Verification items for the finished model (mm, model axes). Give positions to 0.01 mm unless a question says otherwise; leave off trailing zeros. Write each loop counter-clockwise with the first axis right and the second up, starting at its lowest first coordinate (ties: lowest second). Pieces come first, ordered by that corner, then holes.
from build123d import *

# Parameters (mm, degrees)
PAD012_DEPTH = 110
BOX_W        = 174
BOX_H        = 120
BOX_DEPTH    = 10


with BuildPart() as pad012:
    # Sketch015 → Pad012 (new body)
    with BuildSketch(Plane.XZ.offset(-110)):
        Polygon((10, 12.723166), (9.966702, 8.484643), (4.563902, 8.484643), (4.5972, 2), (175.457199, 2.027261), (175.44223, 8.564159), (169.985031, 8.536898), (170, 13), align=None)
    extrude(amount=PAD012_DEPTH)


with BuildPart() as pcb_holder:
    # Box → Box (new body)
    with BuildSketch(Plane(origin=(3, 0, 0), x_dir=(1, 0, 0), z_dir=(0, 0, 1))):
        with Locations((87, 60)):
            Rectangle(BOX_W, BOX_H)
    extrude(amount=BOX_DEPTH)

    # Cut003: cut Pad012
    add(pad012.part, mode=Mode.SUBTRACT)


with BuildPart() as pcb_holder_1:
    # Cut003 placement: moved
    add(pcb_holder.part.moved(Location((0, -1, 0))))


solid = pcb_holder_1.part
Item 1: Release check for a two-part mould opening along Z. For faces 1 (the face through (89.6, -1, 1.6)), 2 (the face through (7, 55, 8.485)), 3 (the face through (89, 60, 0)) record: released by +Z, released by -Z, zero draft, split by the parting line, or undercut.
Answer key:
face 1: zero draft
face 2: undercut
face 3: released by -Z
Item 2: Sectioned sample at B-B on x = 43. Record the cut outline in (y, z).
Answer key:
outline: (-1, 0) - (119, 0) - (119, 10) - (109, 10) - (109, 2.01) - (-1, 2.01) - close
Item 3: Sectioned sample at C-C on z = 6.5. Record the cut outline in (x, y), then the cut area to 3 significant figures.
Answer key:
outline: (3, -1) - (4.57, -1) - (4.57, 109) - (175.45, 109) - (175.45, -1) - (177, -1) - (177, 119) - (3, 119) - close
area: 2,080 mm2
Item 4: Scan lines: line 1 along X through (y, z) = (81.5, 5.25); line 2 along X through (y, z) = (64, 3.25); line 3 along Y through (x, z) = (28, 3.25). Record each from-to range of solid material in increasing order.
Answer key:
line 1: x = 3 to 4.58, 175.45 to 177
line 2: x = 3 to 4.59, 175.45 to 177
line 3: y = 109 to 119
Item 5: Depth check by flat-ended pin: pin 1 (1 mm diameter, centred on x = 153, z = 3.5, fed in from -Y); pin 2 (12 mm diameter, centred on x = 145, y = 28, fed in from +Z). Enter the tip coordinate at first touch or a pass-through.
Answer key:
pin 1: stops at y = 109
pin 2: stops at z = 2.02
Item 6: Sectioned sample at D-D on x = 145. Record the cut outline in (y, z), then the cut area to 3 significant figures.
Answer key:
outline: (-1, 0) - (119, 0) - (119, 10) - (109, 10) - (109, 2.02) - (-1, 2.02) - close
area: 322 mm2
Item 7: Sectioned sample at A-A on y = 102. Record the cut outline in (x, z), then the cut area to 3 significant figures.
Answer key:
outline: (3, 0) - (177, 0) - (177, 10) - (169.99, 10) - (169.99, 8.54) - (175.44, 8.56) - (175.46, 2.03) - (4.6, 2) - (4.56, 8.48) - (9.97, 8.48) - (9.98, 10) - (3, 10) - close
area: 391 mm2
